Can you work these out from the drawing? Everything is in mm from the part's minimum corner. Give positions to 0.01 mm unless a question says otherwise; leave off trailing zeros. Loops run counter-clockwise (first coordinate to the right, second up) from the corner with the lowest first, then second, coordinate; pieces in that order, holes last. Notation, with made-up numbers: (85, 29.5) - (111, 29.5) arc R29 cw to (111, 60.5) - close; hole circle Ø2 at (44.25, 67.5). An arc over 180 degrees is marked (long way). Write each question's results on one line, items separated by ' | '. Start each with the question number.
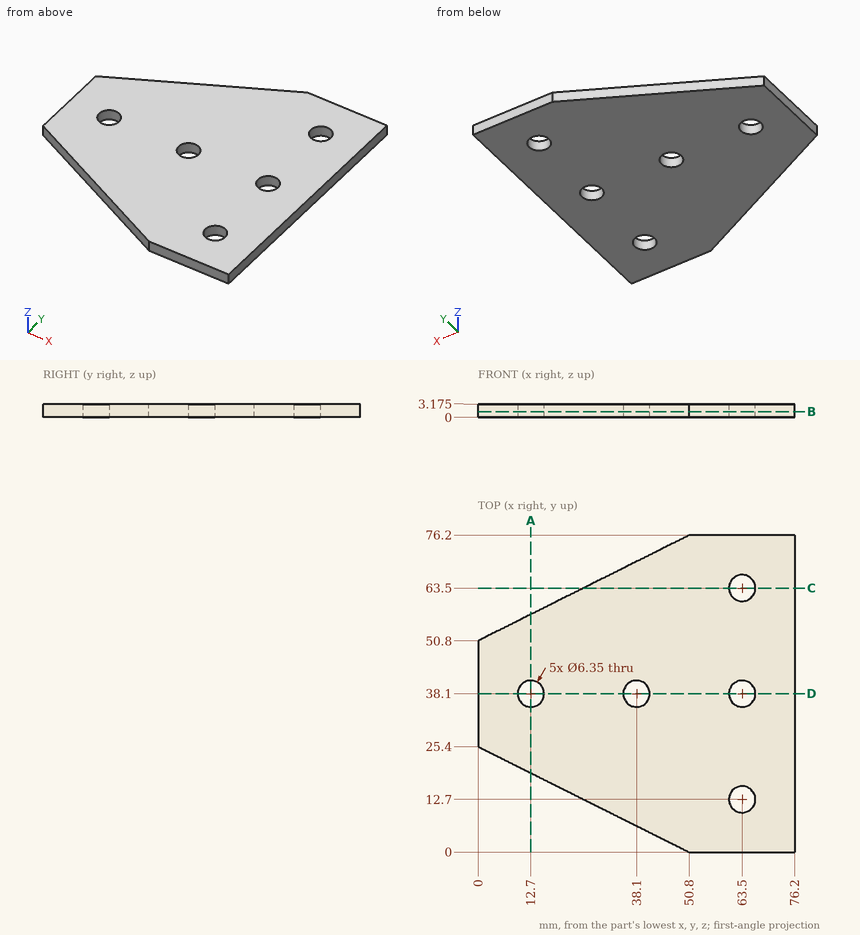
Q1. I want a section at A-A, the plane x = 12.7. List the corners of the cut face in (y, z) for me (3 decimals).
Q2. I want a section at B-B, the plane z = 1.35. List the corners of the cut face in (x, y) for me (3 decimals), then the cut area to 3 significant figures.
Q3. I want a section at D-D, the plane y = 38.1. List the corners of the cut face in (x, z) for me (3 decimals).
Q4. I need wall thicknesses on L1, parallel to Y at x = 63.5, z = 1.5 (3 decimals); L2, parallel to X at y = 36, z = 1.7; L3, parallel to Y at x = 38, z = 2.2. Which ranges of each line are inside material? Lowest first, please. Write a range as from..to.
Q5. I want a section at C-C, the plane y = 63.5. List the corners of the cut face in (x, z) for me (3 decimals), then the cut area to 3 significant figures.
Conclusion:
1) outline: (19.05, 0) - (34.925, 0) - (34.925, 3.175) - (19.05, 3.175) - close; (41.275, 0) - (57.15, 0) - (57.15, 3.175) - (41.275, 3.175) - close
2) outline: (0, 25.4) - (50.8, 0) - (76.2, 0) - (76.2, 76.2) - (50.8, 76.2) - (0, 50.8) - close; hole circle Ø6.35 at (12.7, 38.1); hole circle Ø6.35 at (38.1, 38.1); hole circle Ø6.35 at (63.5, 12.7); hole circle Ø6.35 at (63.5, 38.1); hole circle Ø6.35 at (63.5, 63.5) | area: 4,360 mm^2
3) outline: (0, 0) - (9.525, 0) - (9.525, 3.175) - (0, 3.175) - close; (15.875, 0) - (34.925, 0) - (34.925, 3.175) - (15.875, 3.175) - close; (41.275, 0) - (60.325, 0) - (60.325, 3.175) - (41.275, 3.175) - close; (66.675, 0) - (76.2, 0) - (76.2, 3.175) - (66.675, 3.175) - close
4) L1: 0..9.525, 15.875..34.925, 41.275..60.325, 66.675..76.2 | L2: 0..10.32, 15.08..35.72, 40.48..61.12, 65.88..76.2 | L3: 6.4..34.93, 41.27..69.8
5) outline: (25.4, 0) - (60.325, 0) - (60.325, 3.175) - (25.4, 3.175) - close; (66.675, 0) - (76.2, 0) - (76.2, 3.175) - (66.675, 3.175) - close | area: 141 mm^2
